```python
from build123d import *

# Parameters (mm, degrees)
F0_W         = 121
F0_H         = 195
F1_DEPTH     = 114
F3_DEPTH     = 114
F4_R         = 17
F6_DEPTH     = 134.1
F7_DEPTH     = 135.6
F2_R         = 41
F2_R_2       = 12.5
F8_DEPTH     = 2.8
F9_W         = 71.5012215078
F9_H         = 111.9857653975
F10_DEPTH    = 5
F11_W        = 35
F11_H        = 35
F12_DEPTH    = 35
F13_R        = 15
F14_DEPTH    = 35
F15_T1_DEPTH = 123.1187950266


# Not quite as in the source:
# - a fillet or chamfer that OpenCascade refuses, or shapes differently, is made with other operations: its cross-section is extruded or revolved along the edge and cut away or added


with BuildPart() as f1:
    # F0 (on Right) → F1 (new body)
    with BuildSketch(Plane.YZ):
        with Locations((-7.0141647011, 35.3717551942)):
            Rectangle(F0_W, F0_H)
    extrude(amount=F1_DEPTH)

    # F2 (on face) → F3 (cut, through all)
    with BuildSketch(Plane.YZ.offset(114)):
        Polygon((-60.2907269257, 126.0077205761), (-7.0141647011, 132.8717551942), (-67.5141647011, 132.8717551942), (-67.5141647011, 26.0932128876), align=None)
        Polygon((53.4858352989, 132.8717551942), (-7.0141647011, 132.8717551942), (46.2623975235, 126.0077205761), (53.4858352989, 26.0932128876), align=None)
        Polygon((-62.1019659576, -45.638720619), (-67.5141647011, 26.0932128876), (-67.5141647011, -62.1282448058), (53.4858352989, -62.1282448058), (53.4858352989, 26.0932128876), (48.0736365554, -45.638720619), (-7.0141647011, -49.6213585138), align=None)
    extrude(amount=-F3_DEPTH, mode=Mode.SUBTRACT)

    # F4
    f4_edges = [f1.edges().sort_by_distance(p)[0] for p in [
        (57, -60.290727, 126.007721),
        (57, 46.262398, 126.007721),
        (57, 48.073637, -45.638721),
        (57, -62.101966, -45.638721),
    ]]
    fillet(f4_edges, radius=F4_R)

    # F5 (on Front) → F6 (cut)
    with BuildSketch(Plane.XZ):
        Polygon((56.9999999998, 132.8717551942), (-2e-10, 132.8717551942), (-2e-10, 126.6480237246), align=None)
        Polygon((113.9999999999, 132.8717551942), (56.9999999998, 132.8717551942), (113.9999999999, 126.6480237246), align=None)
    extrude(amount=-F6_DEPTH, mode=Mode.SUBTRACT)

    # F5 (on Front) → F7 (cut)
    with BuildSketch(Plane.XZ):
        Polygon((56.9999999998, 132.8717551942), (-2e-10, 132.8717551942), (-2e-10, 126.6480237246), align=None)
        Polygon((113.9999999999, 132.8717551942), (56.9999999998, 132.8717551942), (113.9999999999, 126.6480237246), align=None)
    extrude(amount=F7_DEPTH, mode=Mode.SUBTRACT)

    # F2 (on face) → F8 (cut)
    with BuildSketch(Plane.YZ.offset(114)):
        with Locations((-7.0141647011, 19.9736393988)):
            Circle(F2_R)
        with Locations((-7.0141647011, 94.7317257524)):
            Circle(F2_R_2)
    extrude(amount=-F8_DEPTH, mode=Mode.SUBTRACT)

    # F9 (on face) → F10 (join)
    with BuildSketch(Plane(origin=(0, 0, 0), x_dir=(0, -1, 0), z_dir=(-1, 0, 0))):
        with Locations((7.0141647011, 18.3268077672)):
            Rectangle(F9_W, F9_H)
    extrude(amount=F10_DEPTH)

    # F11 (on face) → F12 (join)
    with BuildSketch(Plane(origin=(-5, 0, 0), x_dir=(0, -1, 0), z_dir=(-1, 0, 0))):
        with Locations((7.0141647011, 18.3268077672)):
            Rectangle(F11_W, F11_H)
    extrude(amount=F12_DEPTH)

    # F13 (on face) → F14 (cut, through all)
    with BuildSketch(Plane.XY.offset(35.8268077672)):
        with Locations((-22.5, -7.0141647011)):
            Circle(F13_R)
    extrude(amount=-F14_DEPTH, mode=Mode.SUBTRACT)

    # F15: fillet of radius 17.6237590053 on 2 edges, made by hand

    # F15_s2 → F15_t1 (cut)
    with BuildSketch(Plane.XY.offset(-43.2325897462)):
        with BuildLine():
            ThreePointArc((-22.3762409947, -24.5141647011), (-34.8381204973, -19.3522851984), (-40, -6.8904056958))
            Line((-40, -6.8904056958), (-40, -24.5141647011))
            Line((-40, -24.5141647011), (-22.3762409947, -24.5141647011))
        make_face()
        with BuildLine():
            ThreePointArc((-22.3762409947, 10.4858352989), (-34.8381204973, 5.3239557962), (-40, -7.1379237064))
            Line((-40, -7.1379237064), (-40, 10.4858352989))
            Line((-40, 10.4858352989), (-22.3762409947, 10.4858352989))
        make_face()
    extrude(amount=F15_T1_DEPTH, mode=Mode.SUBTRACT)


solid = f1.part
```
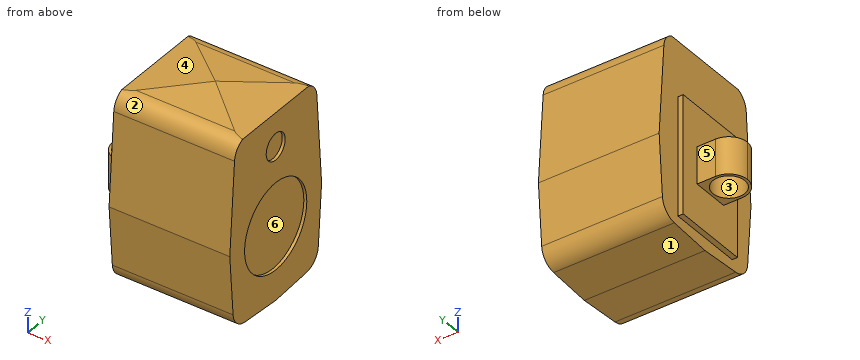
CAD build for the part. Positions are in the model's coordinates, mm. Face numbers are marked on the shaded views. A direction names the side the tool comes from. Coordinates: 2 decimals unless noted, no trailing zeros. Loops run counter-clockwise (first coordinate to the right, second up) from the corner with the lowest first, then second, coordinate; pieces in that order, holes last. Notation, with made-up numbers: (-33.75, -20) - (9.25, -20) arc R20 cw to (9.25, -3) - close; hole circle Ø7 at (79, 24.5). An arc over 180 degrees is marked (long way). Use CSV: the item, a comma, the result in double quotes. Start each with the question number.
Q1. Two-plate mould, pull along Y, no slides. Class the marked faces 1, 2 and 3: +Y half, -Y half, draft (parallel to the pull), parting line (faces both ways), or undercut.
Q2. 3-axis set-ups, long thin cutter, end or side, ignore diameter. For the marked faces 4, 5 and 6: which of +Z, -Z, +X, -X, +Y, -Y reach the whole face in a straight line?
Q3. Drop flat-ended pins along their axis: P1, Ø18, axis at x = -22.5, y = -7.01, coming from the +Z side; P2, Ø3, axis at y = -46, z = 69.5, coming from the -X side; P3, Ø6, axis at x = 93.5, z = -28.5, coming from the -Y side; P4, Ø5, axis at y = -7.5, z = -15.5, coming from the -X side. Give the stop position or say it passes through.
Q4. Cut at A-A, the plane z = 44.5. List the corners of the cut face in (x, y), then the cut area to 3 significant figures.
Q5. Cut at B-B, the plane y = -1.5. List the corners of the cut face in (x, z).
Q6. Probe probe 1 along X at (y, z) = (-8, 31.5); probe 2 along Y at (x, z) = (-22, 22); probe 3 along X at (y, z) = (-57, 25.5). List the from-to ranges inside material, lowest first. Write a range as from..to.
Q7. Cut at D-D, the plane z = -25.5. List the corners of the cut face in (x, y), then the cut area to 3 significant figures.
Q8. Cut at C-C, the plane x = 46. List the corners of the cut face in (y, z), then the cut area to 3 significant figures.
Here are the results:
1,face 1,"+Y half"
1,face 2,"-Y half"
1,face 3,"undercut"
2,face 4,"+Z, -X, +Y, -Y"
2,face 5,"+Z, -Z, -X, +Y"
2,face 6,"+X"
3,P1,"through"
3,P2,"x = 0"
3,P3,"y = -63.62"
3,P4,"x = -5"
4,outline,"(-5, -42.76) - (0, -42.76) - (0, -66.18) - (114, -66.18) - (114, -39.87) - (111.2, -39.87) - (111.2, 25.84) - (114, 25.84) - (114, 52.16) - (0, 52.16) - (0, 28.74) - (-5, 28.74) - close"
4,area,"13,700 mm2"
5,outline,"(-39.07, 0.83) - (-36.45, 0.83) - (-36.45, 35.83) - (-39.07, 35.83) - close; (-8.55, 0.83) - (-5, 0.83) - (-5, -37.67) - (0, -37.67) - (0, -49.22) - (114, -49.22) - (114, -20.65) - (111.2, -20.65) - (111.2, 60.6) - (114, 60.6) - (114, 83.51) - (111.2, 83.51) - (111.2, 105.95) - (114, 105.95) - (114, 126.65) - (63.51, 132.16) - (50.49, 132.16) - (0, 126.65) - (0, 74.32) - (-5, 74.32) - (-5, 35.83) - (-8.55, 35.83) - close"
6,probe 1,"-39.97..-37.47, -7.53..111.2"
6,probe 2,"-24.51..-22.01, 7.98..10.49"
6,probe 3,"0..114"
7,outline,"(-5, -42.76) - (0, -42.76) - (0, -63.62) - (114, -63.62) - (114, 49.59) - (0, 49.59) - (0, 28.74) - (-5, 28.74) - close"
7,area,"13,300 mm2"
8,outline,"(-67.51, 26.09) - (-63.21, -31.02) arc R17 ccw to (-47.48, -46.7) - (-7.01, -49.62) - (33.45, -46.7) arc R17 ccw to (49.18, -31.02) - (53.49, 26.09) - (47.26, 112.15) arc R17 ccw to (32.48, 127.78) - (2.31, 131.67) - (-16.34, 131.67) - (-46.51, 127.78) arc R17 ccw to (-61.29, 112.15) - close"
8,area,"20,100 mm2"
